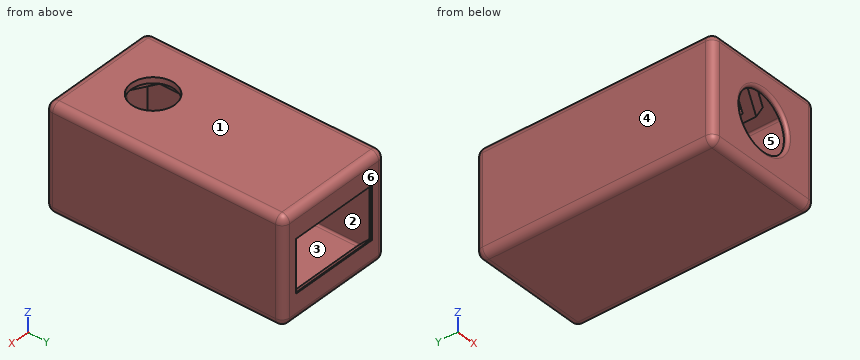
```python
from build123d import *

# Parameters (mm, degrees)
PROFILE_SKETCH_W                         = 55
PROFILE_SKETCH_H                         = 125
PROFILE_EXTRUDE_DEPTH                    = 31.75
INTERIOR_START                           = -3
INTERIOR_SKETCH_W                        = 57.5
INTERIOR_SKETCH_H                        = 49
INTERIOR_CUT_DEPTH                       = 121.4
POWER_SWITCH_OPENING_CUT_REACH           = 142.207
OPENING_SKETCH_W                         = 47.5
OPENING_SKETCH_H                         = 27.4
INSIDE_TOP_CHAMFER_1_SIZE                = 5
INSIDE_TOP_CHAMFER_2_SIZE                = 10.8
STOP_BUTTON_HOLE_CUT_REACH               = 142.207
STOP_BUTTON_HOLE_SKETCH_R                = 11.375
NUT_START                                = -3
NUT_RECESS_EXTRUDE_DEPTH                 = 3
INSIDE_FILLETS_R                         = 1
WIRE_OUTLET_CUT_REACH                    = 142.207
WIRE_OUTLET_CUT_SKETCH_R                 = 15
NUT_RECESS_CHAMFER_FOR_PRINTABILITY_SIZE = 3
WIRE_OUTLET_FILLET_R                     = 1.5
TOP_FILLETS_R                            = 4


# Some blends are built 0.0001 mm under size
with BuildPart() as part:
    # Profile Sketch → Profile Extrude (new, symmetric)
    with BuildSketch(Plane(origin=(0, 0, 0), x_dir=(0, 0, -1), z_dir=(1, 0, 0))):
        with Locations((27.5, 62.5)):
            Rectangle(PROFILE_SKETCH_W, PROFILE_SKETCH_H)
    extrude(amount=PROFILE_EXTRUDE_DEPTH, both=True)

    # Interior Sketch → Interior Cut (cut)
    with BuildSketch(Plane.XZ.offset(INTERIOR_START)):
        with Locations((0, -27.5)):
            Rectangle(INTERIOR_SKETCH_W, INTERIOR_SKETCH_H)
    extrude(amount=-INTERIOR_CUT_DEPTH, mode=Mode.SUBTRACT)

    # Opening Sketch → Power Switch Opening Cut (cut, up to next)
    with BuildSketch(Plane(origin=(0, 125, 0), x_dir=(1, 0, 0), z_dir=(0, 1, 0)), mode=Mode.PRIVATE) as power_switch_opening_cut_sk1:
        with Locations((0, 27.5)):
            Rectangle(OPENING_SKETCH_W, OPENING_SKETCH_H)
    power_switch_opening_cut_tool1 = extrude(power_switch_opening_cut_sk1.sketch, amount=-POWER_SWITCH_OPENING_CUT_REACH, mode=Mode.PRIVATE) & part.part
    add(power_switch_opening_cut_tool1.solids().sort_by_distance((0, 125, -27.5))[0], mode=Mode.SUBTRACT)

    # Inside Top Chamfer 1
    # the kernel refuses this chamfer: 5 mm, written as the material it adds along each edge
    with BuildSketch(Plane(origin=(28.75, 124.4, -52), x_dir=(-0.9996219169112968, 0.0274958766105877, 0), z_dir=(0, 0, 1)), Plane(origin=(-28.75, 124.4, -3), x_dir=(0.9996219169112968, 0.0274958766105877, 0), z_dir=(0, 0, -1))) as inside_top_chamfer_1_piece_1:
        Polygon((INSIDE_TOP_CHAMFER_1_SIZE * 0.999621916911, INSIDE_TOP_CHAMFER_1_SIZE * 0.0274958766106), (-INSIDE_TOP_CHAMFER_1_SIZE * 0.0274958766106, INSIDE_TOP_CHAMFER_1_SIZE * 0.999621916911), (0, 0), align=None)
    extrude(amount=49)

    # Inside Top Chamfer 2
    inside_top_chamfer_2_edges = [part.edges().sort_by_distance(p)[0] for p in [
        (0, 124.4, -52),
        (0, 124.4, -3),
    ]]
    chamfer(inside_top_chamfer_2_edges, length=INSIDE_TOP_CHAMFER_2_SIZE - 0.0001)  # a hair under: the kernel refuses the full size

    # Stop Button Hole Sketch → Stop Button Hole Cut (cut, up to next)
    with BuildSketch(Plane.XY, mode=Mode.PRIVATE) as stop_button_hole_cut_sk1:
        with Locations((0, 30)):
            Circle(STOP_BUTTON_HOLE_SKETCH_R)
    stop_button_hole_cut_tool1 = extrude(stop_button_hole_cut_sk1.sketch, amount=-STOP_BUTTON_HOLE_CUT_REACH, mode=Mode.PRIVATE) & part.part
    add(stop_button_hole_cut_tool1.solids().sort_by_distance((0, 30, 0))[0], mode=Mode.SUBTRACT)

    # Stop Button Nut Sketch → Nut Recess Extrude (add)
    with BuildSketch(Plane.XY.offset(NUT_START)):
        Polygon((0, 8.926715175), (18.25, 19.463357587), (18.25, 40.536642413), (0, 51.073284825), (-18.25, 40.536642413), (-18.25, 19.463357587), align=None)
        Polygon((-13.25, 22.350108933), (0, 14.700217866), (13.25, 22.350108933), (13.25, 37.649891067), (0, 45.299782134), (-13.25, 37.649891067), align=None, mode=Mode.SUBTRACT)
    extrude(amount=-NUT_RECESS_EXTRUDE_DEPTH)

    # Inside Fillets
    inside_fillets_edges = [part.edges().sort_by_distance(p)[0] for p in [
        (28.75, 58.30005, -52),
        (-28.75, 58.30005, -52),
        (-28.75, 58.30005, -3),
        (28.75, 58.30005, -3),
    ]]
    fillet(inside_fillets_edges, radius=INSIDE_FILLETS_R)

    # Wire Outlet Cut Sketch → Wire Outlet Cut (cut, up to next)
    with BuildSketch(Plane.XZ, mode=Mode.PRIVATE) as wire_outlet_cut_sk1:
        with Locations(Location((0, -27.5, 0), (0, 0, 270))):
            Circle(WIRE_OUTLET_CUT_SKETCH_R)
    wire_outlet_cut_tool1 = extrude(wire_outlet_cut_sk1.sketch, amount=-WIRE_OUTLET_CUT_REACH, mode=Mode.PRIVATE) & part.part
    add(wire_outlet_cut_tool1.solids().sort_by_distance((0, 0, -27.5))[0], mode=Mode.SUBTRACT)

    # Nut Recess Chamfer for Printability
    nut_recess_chamfer_for_printability_edges = [part.edges().sort_by_distance(p)[0] for p in [
        (9.125, 14.195036381, -3),
        (-9.125, 14.195036381, -3),
    ]]
    chamfer(nut_recess_chamfer_for_printability_edges, length=NUT_RECESS_CHAMFER_FOR_PRINTABILITY_SIZE - 0.0001)  # a hair under: the kernel refuses the full size

    # Wire Outlet Fillet
    wire_outlet_fillet_edges = [part.edges().sort_by_distance(p)[0] for p in [
        (0, 0, -12.5),
        (0, 3, -12.5),
    ]]
    fillet(wire_outlet_fillet_edges, radius=WIRE_OUTLET_FILLET_R - 0.0001)  # a hair under: the kernel refuses the full size

    # Top Fillets
    top_fillets_edges = [part.edges().sort_by_distance(p)[0] for p in [
        (31.75, 125, -27.5),
        (31.75, 62.5, 0),
        (31.75, 0, -27.5),
        (-31.75, 62.5, 0),
        (-31.75, 125, -27.5),
        (-31.75, 62.5, -55),
        (-31.75, 0, -27.5),
        (0, 0, 0),
        (0, 125, 0),
        (0, 125, -55),
        (0, 0, -55),
        (31.75, 62.5, -55),
    ]]
    fillet(top_fillets_edges, radius=TOP_FILLETS_R)


solid = part.part
```
Input: part model. Units: mm. Frame: model coordinates. Face numbers are marked on the shaded views. A direction names the side the tool comes from. Give positions to 0.01 mm unless a question says otherwise; leave off trailing zeros. Order: outer loops, then holes, each group sorted by start corner. A loop starts at its lowest first (then second) coordinate and runs counter-clockwise, first axis right, second up.
1. Section D-D on y = 30. Return the cut outline in (x, z) (3 decimals), and give its area (3 significant figures).
Derived:
outline: (-31.75, -51) arc R4 ccw to (-27.75, -55) - (27.75, -55) arc R4 ccw to (31.75, -51) - (31.75, -4) arc R4 ccw to (27.75, 0) - (11.375, 0) - (11.375, -3) - (13.25, -3) - (13.25, -6) - (18.25, -6) - (18.25, -3) - (27.75, -3) arc R1 cw to (28.75, -4) - (28.75, -51) arc R1 cw to (27.75, -52) - (-27.75, -52) arc R1 cw to (-28.75, -51) - (-28.75, -4) arc R1 cw to (-27.75, -3) - (-18.25, -3) - (-18.25, -6) - (-13.25, -6) - (-13.25, -3) - (-11.375, -3) - (-11.375, 0) - (-27.75, 0) arc R4 ccw to (-31.75, -4) - close
area: 624 mm2
2. Section C-C on x = 25. Return the cut outline in (y, z).
Derived:
outline: (0, -51) arc R4 ccw to (4, -55) - (121, -55) arc R4 ccw to (125, -51) - (125, -4) arc R4 ccw to (121, 0) - (4, 0) arc R4 ccw to (0, -4) - close; hole (3, -52) - (113.6, -52) - (123.15, -42.45) - (123.15, -12.55) - (113.6, -3) - (3, -3) - close
3. Pin query (flat end, axial travel): pin 1 (0.7 mm diameter, centred on x = -3, y = 124.5, fed in from +Z); pin 2 (6 mm diameter, centred on x = 18.5, z = -20, fed in from +Y). Return the tip coordinate at first contact, or that it passes through.
Derived:
pin 1: stops at z = -1.53
pin 2: stops at y = 3
4. Section B-B on y = 98. Return the cut outline in (x, z), and give its area (3 significant figures).
Derived:
outline: (-31.75, -51) arc R4 ccw to (-27.75, -55) - (27.75, -55) arc R4 ccw to (31.75, -51) - (31.75, -4) arc R4 ccw to (27.75, 0) - (-27.75, 0) arc R4 ccw to (-31.75, -4) - close; hole (-28.75, -51) arc R1 ccw to (-27.75, -52) - (27.75, -52) arc R1 ccw to (28.75, -51) - (28.75, -4) arc R1 ccw to (27.75, -3) - (-27.75, -3) arc R1 ccw to (-28.75, -4) - close
area: 662 mm2
5. Material intervals for L1, parallel to Z at x = -13.5, y = 90; L2, parallel to X at y = 76, z = -34; L3, parallel to Y at x = 17.5, z = -20.5, sorted ascending.
Derived:
L1: z = -55 to -52, -3 to 0
L2: x = -31.75 to -28.75, 28.75 to 31.75
L3: y = 0 to 3
6. Reachability of the marked faces 5 and 6 from +Z, -Z, +X, -X, +Y, -Y: full face, straight path, thin tool, end or side. Return the list, or none.
Derived:
face 5: none
face 6: +Z, -Z, +X, -X, +Y
7. Mould query, pull axis X, two halves, no side actions, for the marked faces 1, 2, 3 and 4. Classes: released by +X, released by -X, zero draft, split by the parting line, or undercut.
Derived:
face 1: zero draft
face 2: undercut
face 3: undercut
face 4: released by -X
